Can you work these out from the drawing? Everything is in mm from the part's minimum corner. Give positions to 0.01 mm unless a question says otherwise; leave off trailing zeros. Write each loop counter-clockwise with the first axis right and the second up, starting at its lowest first coordinate (ties: lowest second). Pieces come first, ordered by that corner, then holes. Notation, with made-up numbers: (-34.75, -1.75) -> (-20.75, -1.75) arc R14 cw to (-20.75, 16.25) -> close; hole circle Ø3 at (66.5, 7.5). An arc over 180 degrees is marked (long way). Use one line per item in the form item = value.
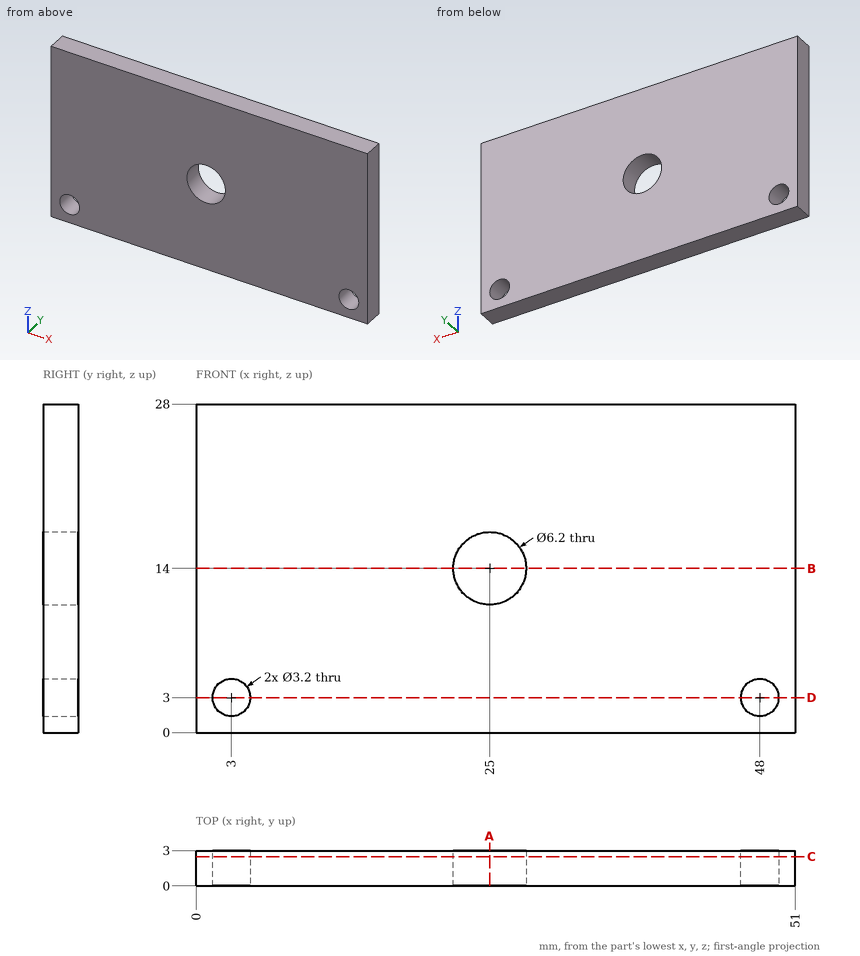
Q1. I want a section at A-A, the plane x = 25. Write out the boundary of the cut face in (y, z), and give its area (3 significant figures).
Result set:
outline = (0, 0) -> (3, 0) -> (3, 10.9) -> (0, 10.9) -> close; (0, 17.1) -> (3, 17.1) -> (3, 28) -> (0, 28) -> close
area = 65.4 mm2
Q2. I want a section at C-C, the plane y = 2.5. Write out the boundary of the cut face in (x, z).
Result set:
outline = (0, 0) -> (51, 0) -> (51, 28) -> (0, 28) -> close; hole circle Ø3.2 at (3, 3); hole circle Ø6.2 at (25, 14); hole circle Ø3.2 at (48, 3)
Q3. If I drill on line 1 along X through (y, z) = (1.6, 3); line 2 along X through (y, z) = (2.2, 14); line 3 along Z through (x, y) = (48, 1.45), over which ranges is the centre line in solid material (lowest first)? Write a range as from..to.
Result set:
line_1 = 0..1.4, 4.6..46.4, 49.6..51
line_2 = 0..21.9, 28.1..51
line_3 = 0..1.4, 4.6..28
Q4. I want a section at B-B, the plane z = 14. Write out the boundary of the cut face in (x, y).
Result set:
outline = (0, 0) -> (21.9, 0) -> (21.9, 3) -> (0, 3) -> close; (28.1, 0) -> (51, 0) -> (51, 3) -> (28.1, 3) -> close
Q5. Will this pin go through, and if not, where does the flat tip stop? pin 1 Ø3 at (x, z) = (48, 3) entering from +Y.
Result set:
pin_1 = through
Q6. I want a section at D-D, the plane z = 3. Write out the boundary of the cut face in (x, y).
Result set:
outline = (0, 0) -> (1.4, 0) -> (1.4, 3) -> (0, 3) -> close; (4.6, 0) -> (46.4, 0) -> (46.4, 3) -> (4.6, 3) -> close; (49.6, 0) -> (51, 0) -> (51, 3) -> (49.6, 3) -> close
